Check sheet for the modelled part. Datum: model origin and axes. Units: mm. A direction names the side the tool comes from. Give positions to 0.01 mm unless a question says otherwise; leave off trailing zeros. Order: outer loops, then holes, each group sorted by start corner. A loop starts at its lowest first (then second) coordinate and runs counter-clockwise, first axis right, second up.
from build123d import *

# Parameters (mm, degrees)
SKETCH1_R           = 76.2
BOSS_EXTRUDE1_DEPTH = 38.1


with BuildPart() as part:
    # Sketch1 → Boss-Extrude1 (new body)
    with BuildSketch(Plane.XY):
        Circle(SKETCH1_R)
        with BuildLine():
            ThreePointArc((9.5377, 0), (-5.502926267, -7.790091385), (-3.1877, 8.989231892))
            Line((-3.1877, 8.989231892), (-3.1877, 12.7254))
            Line((-3.1877, 12.7254), (3.1877, 12.7254))
            Line((3.1877, 12.7254), (3.1877, 8.989231892))
            ThreePointArc((3.1877, 8.989231892), (7.790091385, 5.502926267), (9.5377, 0))
        make_face(mode=Mode.SUBTRACT)
    extrude(amount=BOSS_EXTRUDE1_DEPTH)


solid = part.part
1) Section check A-A, the plane x = 0. Record the cut outline in (y, z).
Recorded:
outline: (-76.2, 0) - (-9.54, 0) - (-9.54, 38.1) - (-76.2, 38.1) - close; (12.73, 0) - (76.2, 0) - (76.2, 38.1) - (12.73, 38.1) - close
2) Material ranges on L1, parallel to Y at x = 0, z = 24.5; L2, parallel to Y at x = 52.5, z = 18.5; L3, parallel to X at y = 44, z = 14.5, recorded low to high.
Recorded:
L1: y = -76.2 to -9.54, 12.73 to 76.2
L2: y = -55.23 to 55.23
L3: x = -62.21 to 62.21
3) Section check C-C, the plane y = 4.5. Record the cut outline in (x, z).
Recorded:
outline: (-76.07, 0) - (-8.41, 0) - (-8.41, 38.1) - (-76.07, 38.1) - close; (8.41, 0) - (76.07, 0) - (76.07, 38.1) - (8.41, 38.1) - close
4) Section check B-B, the plane z = 14.5. Record the cut outline in (x, y), then the cut area to 3 significant figures.
Recorded:
outline: circle Ø152.4 at (0, 0); hole (-3.19, 8.99) arc R9.54 ccw (long way) to (3.19, 8.99) - (3.19, 12.73) - (-3.19, 12.73) - close
area: 17,900 mm2
5) Section check D-D, the plane y = -56. Record the cut outline in (x, z), then the cut area to 3 significant figures.
Recorded:
outline: (-51.68, 0) - (51.68, 0) - (51.68, 38.1) - (-51.68, 38.1) - close
area: 3,940 mm2
6) Depth check by flat-ended pin: pin 1 Ø1.1 at (y, z) = (11, 19) entering from +X; pin 2 Ø1 at (x, z) = (-3.5, 23.5) entering from +Y; pin 3 Ø5 at (x, z) = (1, 18) entering from -Y. Enter the tip coordinate at first touch or a pass-through.
Recorded:
pin 1: stops at x = 75.48
pin 2: stops at y = 76.14
pin 3: stops at y = -76.2
7) Set-up check for faces 1 (the face through (16, 1, 38.1)), 2 (the face through (0, 12.725, 19)): record each of +Z, -Z, +X, -X, +Y, -Y from which the full face is reachable in a straight line by a thin tool's end or side.
Recorded:
face 1: +Z, +X, -X, +Y, -Y
face 2: +Z, -Z
8) Draft check along X on faces 3 (the face through (16, 1, 0)), 4 (the face through (-3.188, 11, 19)), 5 (the face through (-60.47, -46.367, 18.783)). Enter one of: +X half, -X half, draft (parallel to the pull), parting line (faces both ways), or undercut.
Recorded:
face 3: draft
face 4: undercut
face 5: parting line
